Design review of the part shown in the three views and the two pictorial views. Dimensions are in mm from the part's minimum x, y and z. A direction names the side the tool comes from. Coordinates: 2 decimals unless noted, no trailing zeros. Loops run counter-clockwise (first coordinate to the right, second up) from the corner with the lowest first, then second, coordinate; pieces in that order, holes last. Notation, with made-up numbers: (67, 32.5) - (76, 32.5) arc R17 cw to (76, 56.5) - close; hole circle Ø10 at (37, -16.75). An arc over 180 degrees is marked (long way). One line per item, written item: value. Start each with the question number.
1. For the marked faces 1, 2 and 3, list the 3-axis set-ups (+Z, -Z, +X, -X, +Y, -Y) from which the entire face can be reached by the end or side of a thin tool; tool diameter is ignored.
2. Take a section at C-C, the plane z = 10.25. State the section outline as (x, y) points (1 decimal).
3. Take a section at D-D, the plane y = 23.75. State the section outline as (x, z) points.
4. Take a section at A-A, the plane x = 38.5. State the section outline as (y, z) points (1 decimal), and give its area (3 significant figures).
5. Insertion check: pin 1 (1.5 mm diameter, centred on y = 5.5, z = 17.5, fed in from -X); pin 2 (4 mm diameter, centred on x = 10, y = 20.5, fed in from +Z); pin 3 (6 mm diameter, centred on x = 37, z = 11.5, fed in from +Y) (1 decimal); pin 4 (4 mm diameter, centred on x = 35.5, y = 22, fed in from +Z). Each pin has a flat end and moves straight along its axis. Give the tip position at first contact, or say it passes through.
6. To check wall thickness, follow line 1 (Z direction, x = 10, y = 7.5) (1 decimal); line 2 (Z direction, x = 4.5, y = 12.5); line 3 (X direction, y = 17, z = 23). State the ranges of each line that lie inside material, in increasing order. Write a range as from..to.
7. Take a section at B-B, the plane y = 8.25. State the section outline as (x, z) points.
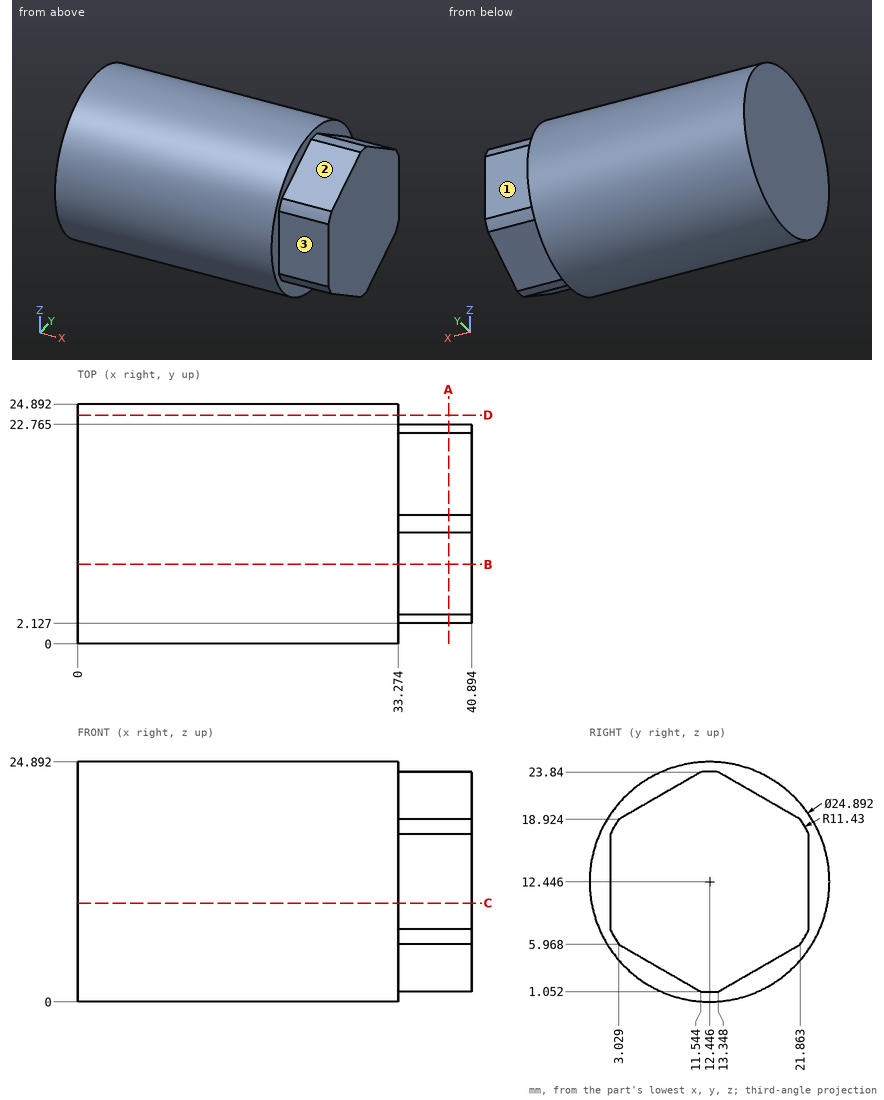
Solutions:
1. face 1: +Z, -Z, +X, +Y
1. face 2: +Z, +X, -Y
1. face 3: +Z, -Z, +X, -Y
2. outline: (0, 0.2) - (33.3, 0.2) - (33.3, 2.1) - (40.9, 2.1) - (40.9, 22.8) - (33.3, 22.8) - (33.3, 24.7) - (0, 24.7) - close
3. outline: (0, 7.24) - (33.27, 7.24) - (33.27, 17.65) - (0, 17.65) - close
4. outline: (2.1, 7.5) arc R11.4 ccw to (3, 6) - (11.5, 1.1) arc R11.4 ccw to (13.3, 1.1) - (21.9, 6) arc R11.4 ccw to (22.8, 7.5) - (22.8, 17.4) arc R11.4 ccw to (21.9, 18.9) - (13.3, 23.8) arc R11.4 ccw to (11.5, 23.8) - (3, 18.9) arc R11.4 ccw to (2.1, 17.4) - close
4. area: 366 mm2
5. pin 1: x = 0
5. pin 2: z = 23.32
5. pin 3: y = 22.8
5. pin 4: z = 20
6. line 1: 1..23.9
6. line 2: 0..24.89
6. line 3: 0..33.27
7. outline: (0, 0.73) - (33.27, 0.73) - (33.27, 2.95) - (40.89, 2.95) - (40.89, 21.94) - (33.27, 21.94) - (33.27, 24.16) - (0, 24.16) - close
